For this review, take the finished solid that the model builds, in its own axes (mm). Round coordinates to 2 decimals unless told otherwise and drop trailing zeros. Order: outer loops, then holes, each group sorted by start corner. A loop starts at its lowest first (then second) coordinate and runs counter-clockwise, first axis right, second up.
```python
from build123d import *

# Parameters (mm, degrees)
F6_COUNT = 5
F7_COUNT = 2


with BuildPart() as f4:
    # F3 (on line) → F4 section 0
    with BuildSketch(Plane.XY.offset(11.1351636441), mode=Mode.PRIVATE) as f4_s0:
        Polygon((5, 6.8819096024), (-5, 6.8819096024), (-8.0901699437, -2.6286555606), (0, -8.5065080835), (8.0901699437, -2.6286555606), align=None)
    loft([f4_s0.sketch, Vertex(0, 0, 0)])


with BuildPart() as f5_1:
    # F5: instance of F4
    add(f4.part.mirror(Plane(origin=(0, 4.5879397349, 7.4234424294), x_dir=(-1, 0, 0), z_dir=(0, 0.8506508084, -0.5257311121))))


with BuildPart() as f6_1:
    # F6: instance of F5_1
    add(f5_1.part.rotate(Axis((0, 0, 5.5675818221), (0, 0, 1)), 1 * 360 / F6_COUNT))


with BuildPart() as f6_2:
    # F6: instance of F5_1
    add(f5_1.part.rotate(Axis((0, 0, 5.5675818221), (0, 0, 1)), 2 * 360 / F6_COUNT))


with BuildPart() as f6_3:
    # F6: instance of F5_1
    add(f5_1.part.rotate(Axis((0, 0, 5.5675818221), (0, 0, 1)), 3 * 360 / F6_COUNT))


with BuildPart() as f6_4:
    # F6: instance of F5_1
    add(f5_1.part.rotate(Axis((0, 0, 5.5675818221), (0, 0, 1)), 4 * 360 / F6_COUNT))


with BuildPart() as f4_1:
    add(f4.part)

    add(f5_1.part)  # F7 merges F5_1

    add(f6_1.part)  # F7 merges F6_1

    add(f6_2.part)  # F7 merges F6_2

    add(f6_3.part)  # F7 merges F6_3

    add(f6_4.part)  # F7 merges F6_4
    # F7: F4, F6_3, F6_4, F5_1, F6_2, F6_1 ×2 about axis
    f7_axis = Axis((0, 0, 0), (1, 0, 0))
    for i in range(1, F7_COUNT):
        add(f4.part.rotate(f7_axis, i * 360 / F7_COUNT))
        add(f6_3.part.rotate(f7_axis, i * 360 / F7_COUNT))
        add(f6_4.part.rotate(f7_axis, i * 360 / F7_COUNT))
        add(f5_1.part.rotate(f7_axis, i * 360 / F7_COUNT))
        add(f6_2.part.rotate(f7_axis, i * 360 / F7_COUNT))
        add(f6_1.part.rotate(f7_axis, i * 360 / F7_COUNT))


solid = f4_1.part
```
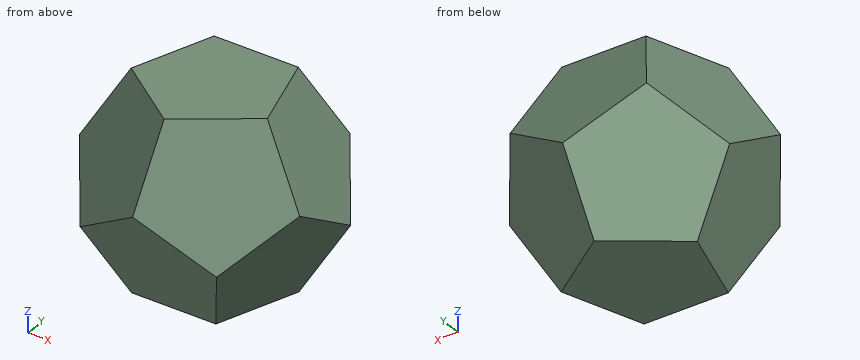
Q1. Wall thickness on line 1 (Y direction, x = 7, z = 0); line 2 (X direction, y = 8.75, z = -1.75); line 3 (Y direction, x = 5.5, z = -9): over which ranges is each line inside the solid? List them lowest first.
Q2. Take a section at A-A, the plane y = -3. State the section outline as (x, z) points.
Q3. Take a section at C-C, the plane z = 1.5. State the section outline as (x, y) points, plus the area to 3 significant figures.
Q4. Take a section at D-D, the plane x = -1.75. State the section outline as (y, z) points.
Q5. Clearance check with flat-ended pins moving along their axes: pin 1 (10 mm diameter, centred on y = -3, z = -3.5, fed in from +X); pin 2 (1 mm diameter, centred on x = -4.5, z = -6.5, fed in from +Y); pin 3 (2 mm diameter, centred on x = 10.5, y = 5, fed in from +Z); pin 4 (6 mm diameter, centred on x = -5, y = -10.5, fed in from -Z). State where each tip first meets the part, or that it passes through.
Q6. Take a section at B-B, the plane x = -6. State the section outline as (y, z) points.
Working result:
1. line 1: y = -10.3 to 10.3
1. line 2: x = -7.65 to 7.65
1. line 3: y = -7.95 to 5.83
2. outline: (-13.09, 1.85) - (-6.26, -11.14) - (6.26, -11.14) - (13.09, 1.85) - (9.23, 9.19) - (7.58, 11.14) - (-7.58, 11.14) - (-9.23, 9.19) - close
3. outline: (-13.09, -2.43) - (-12.02, -5.73) - (-1.74, -13.2) - (1.74, -13.2) - (12.02, -5.73) - (13.09, -2.43) - (9.16, 9.66) - (6.35, 11.7) - (-6.35, 11.7) - (-9.16, 9.66) - close
3. area: 486 mm2
4. outline: (-13.2, 1.49) - (-6.88, -11.14) - (7.24, -11.14) - (13.2, -1.49) - (6.88, 11.14) - (-7.24, 11.14) - close
5. pin 1: stops at x = 13.09
5. pin 2: stops at y = 8.58
5. pin 3: stops at z = 3.84
5. pin 4: stops at z = -9.9
6. outline: (-11.81, -1.27) - (-8.26, -8.38) - (-3.8, -11.14) - (4.15, -11.14) - (11.81, 1.27) - (8.26, 8.38) - (3.8, 11.14) - (-4.15, 11.14) - close
